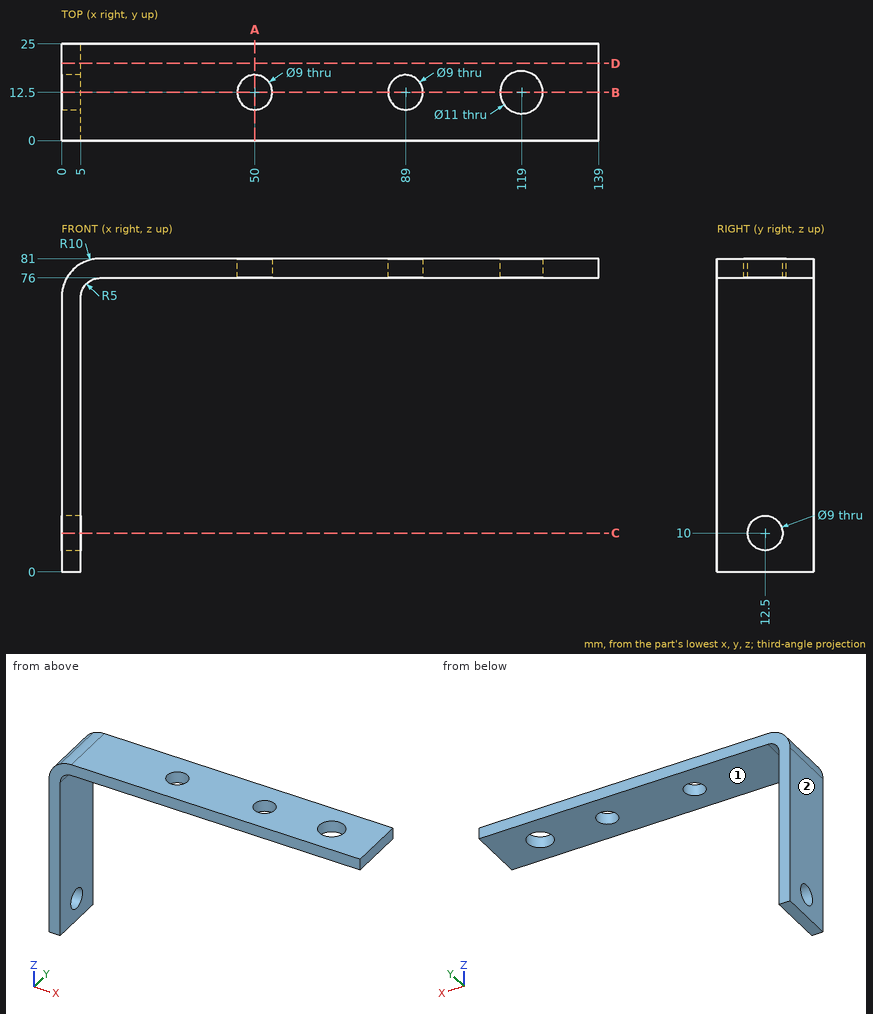
Job drawing, mm, ordinate dimensions from the low corner. One solid piece. A direction names the side the tool comes from. Coordinates: 2 decimals unless noted, no trailing zeros. Write each loop counter-clockwise with the first axis right and the second up, starting at its lowest first coordinate (ties: lowest second). Pieces come first, ordered by that corner, then holes. Notation, with made-up numbers: M -27,80 L 6,80 A18 cw 6,102 Z; hole C -29.5,76.25 d3. An arc over 180 degrees is marked long. Answer as a JSON object with one key per item and string values. Group by question number.
1) Pin check, flat tips, straight feed: pin 1 Ø1.5 at (x, y) = (121, 14.5) entering from -Z; pin 2 Ø3 at (y, z) = (20, 61) entering from +X. Stop position of each tip, or through.
2) Tool access for the marked faces 1 and 2: list every direction of +Z, -Z, +X, -X, +Y, -Y with a clear straight run to the whole face (end or side of a thin tool).
3) Wall check: line 1 (Y direction, x = 89, z = 78); line 2 (Y direction, x = 119, z = 79.75); line 3 (Z direction, x = 28.5, y = 10.5). Give the ranges that are in metal, low to high. Write a range as from..to.
4) Saw through at C-C (z = 10). Write the cut outline in (x, y), plus the area to 3 significant figures.
5) Saw through at D-D (y = 20). Write the cut outline in (x, z).
6) Saw through at B-B (y = 12.5). Write the cut outline in (x, z).
7) Saw through at A-A (x = 50). Write the cut outline in (y, z).
Values follow:
{
 "1": {"pin 1": "passes through", "pin 2": "stops at x = 5"},
 "2": {"face 1": "-Z, +X, +Y, -Y", "face 2": "+Z, -Z, -X, +Y, -Y"},
 "3": {"line 1": "y = 0..8, 17..25", "line 2": "y = 0..7, 18..25", "line 3": "z = 76..81"},
 "4": {"outline": "M 0,0 L 5,0 L 5,8 L 0,8 Z; M 0,17 L 5,17 L 5,25 L 0,25 Z", "area": "80.0 mm2"},
 "5": {"outline": "M 0,0 L 5,0 L 5,71 A5 cw 10,76 L 139,76 L 139,81 L 10,81 A10 ccw 5,79.66 A10 ccw 0,71 Z"},
 "6": {"outline": "M 0,0 L 5,0 L 5,5.5 L 0,5.5 Z; M 0,14.5 L 5,14.5 L 5,71 A5 cw 10,76 L 45.5,76 L 45.5,81 L 10,81 A10 ccw 5,79.66 A10 ccw 0,71 Z; M 54.5,76 L 84.5,76 L 84.5,81 L 54.5,81 Z; M 93.5,76 L 113.5,76 L 113.5,81 L 93.5,81 Z; M 124.5,76 L 139,76 L 139,81 L 124.5,81 Z"},
 "7": {"outline": "M 0,76 L 8,76 L 8,81 L 0,81 Z; M 17,76 L 25,76 L 25,81 L 17,81 Z"}
}
